Work out the finished part from the listing and answer in its coordinate system (mm). Face numbers are marked on the shaded views. Round coordinates to 2 decimals unless told otherwise and drop trailing zeros. Write each loop counter-clockwise with the first axis right and the second up, starting at its lowest first coordinate (ties: lowest second). Pieces come first, ordered by that corner, then holes.
1. Find section A-A (z = 5). Write down the section's boundary in (x, y).
2. Find section B-B (y = -22). Write down the section's boundary in (x, z).
3. Determine the mould class of the marked faces 1, 2 and 3 for opening direction X: pulls with the +X half, pulls with the -X half, needs draft (parallel to the pull), parting line crosses it, or undercut.
4. Find section C-C (x = 0). Write down the section's boundary in (y, z).
5. Flat-ended cylindrical pins translate along their axes: pin 1 Ø6 at (y, z) = (-58, 2) entering from +X; pin 2 Ø3 at (x, y) = (-4.5, -52.5) entering from +Z; pin 3 Ø0.7 at (x, z) = (-5.5, -2) entering from -Y. Find the tip coordinate at first contact, or state that the pin passes through.
6. Straight lines are drawn through the part: probe 1 along Z at (x, y) = (0, -62.25); probe 2 along Z at (x, y) = (0, -67); probe 3 along Z at (x, y) = (0, 7.5). For each, find the intervals that lie inside material, in ascending order.
7. Find section D-D (z = 0). Write down the section's boundary in (x, y).
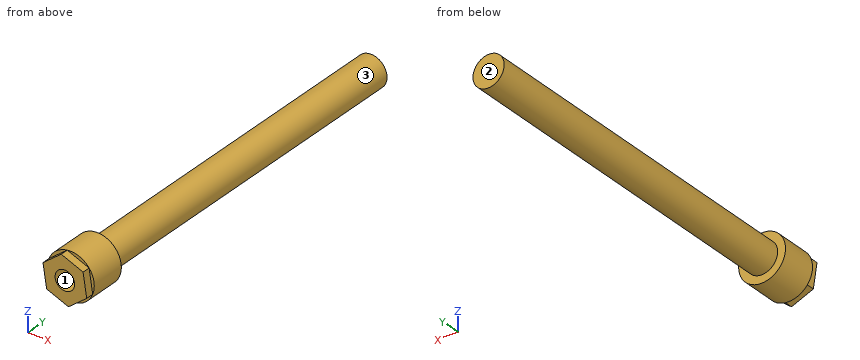
```python
from build123d import *

# Parameters (mm, degrees)
F0_R          = 6
F1_DEPTH      = 75
F1_DEPTH_BACK = 25
F3_DEPTH      = 2
F4_R          = 2.5
F5_DEPTH      = 25
F6_R          = 6
F6_R_2        = 4
F7_DEPTH      = 91


with BuildPart() as f1:
    # F0 (on Front) → F1 (new body, two sides)
    with BuildSketch(Plane.XZ) as f1_sk:
        Circle(F0_R)
    extrude(amount=F1_DEPTH)
    extrude(f1_sk.sketch, amount=-F1_DEPTH_BACK)

    # F2 (on face) → F3 (join)
    with BuildSketch(Plane.XZ.offset(75)):
        Polygon((5.597545, -2.160437), (4.669766, 3.767398), (-0.927779, 5.927835), (-5.597545, 2.160437), (-4.669766, -3.767398), (0.927779, -5.927835), align=None)
    extrude(amount=F3_DEPTH)

    # F4 (on face) → F5 (cut)
    with BuildSketch(Plane.XZ.offset(77)):
        Circle(F4_R)
    extrude(amount=-F5_DEPTH, mode=Mode.SUBTRACT)

    # F6 (on face) → F7 (cut)
    with BuildSketch(Plane(origin=(0, 25, 0), x_dir=(-1, 0, 0), z_dir=(0, 1, 0))):
        Circle(F6_R)
        Circle(F6_R_2, mode=Mode.SUBTRACT)
    extrude(amount=-F7_DEPTH, mode=Mode.SUBTRACT)


solid = f1.part
```
Worked answers:
1. outline: (-3.32, -75) - (-2.08, -75) - (-2.08, -77) - (1.48, -77) - (1.48, -75) - (3.32, -75) - (3.32, -66) - (-3.32, -66) - close
2. outline: circle Ø8 at (0, 0)
3. face 1: undercut
3. face 2: needs draft
3. face 3: parting line crosses it
4. outline: (-77, -5.57) - (-75, -5.57) - (-75, -6) - (-66, -6) - (-66, -4) - (25, -4) - (25, 4) - (-66, 4) - (-66, 6) - (-75, 6) - (-75, 5.57) - (-77, 5.57) - (-77, 2.5) - (-52, 2.5) - (-52, -2.5) - (-77, -2.5) - close
5. pin 1: stops at x = 4
5. pin 2: stops at z = 2.65
5. pin 3: stops at y = -75
6. probe 1: z = -4 to -2.5, 2.5 to 4
6. probe 2: z = -6 to -2.5, 2.5 to 6
6. probe 3: z = -4 to 4
7. outline: (-6, -75) - (-5.26, -75) - (-5.26, -77) - (-2.5, -77) - (-2.5, -52) - (2.5, -52) - (2.5, -77) - (5.26, -77) - (5.26, -75) - (6, -75) - (6, -66) - (4, -66) - (4, 25) - (-4, 25) - (-4, -66) - (-6, -66) - close
